```python
from build123d import *

# Parameters (mm, degrees)
EXTRUDE_373_DEPTH      = 12.5
SKETCH_4_W             = 0.8
SKETCH_4_H             = 12.320508076
CHAMFER_2074_SIZE      = 2
FILLET_2116_R          = 0.8
PATTERN_LINEAR_1_COUNT = 20
PATTERN_LINEAR_1_PITCH = 2.421052632


with BuildPart() as part:
    # 草图1 → Extrude 373 (new body)
    with BuildSketch(Plane(origin=(0, 0, 0), x_dir=(0, 0, -1), z_dir=(1, 0, 0))):
        Polygon((15, 8.660254038), (15, -8.660254038), (0, -17.320508076), (-15, -8.660254038), (-15, 8.660254038), (0, 17.320508076), align=None)
    extrude(amount=EXTRUDE_373_DEPTH)

    # 草图2 → 凸台-旋转1 (revolve)
    with BuildSketch(Plane.XY, mode=Mode.PRIVATE) as revolve_1_sk:
        Polygon((0, 0), (92.5, 0), (92.5, 7.835), (92.5, 10), (27.8072, 10), (0, 10), align=None)
    revolve(revolve_1_sk.sketch.rotate(Axis((0, 0, 0), (1, 0, 0)), 90), axis=Axis((0, 0, 0), (1, 0, 0)))

    # 草图3 → 切除-旋转1 (revolve, cut)
    with BuildSketch(Plane.XY):
        Polygon((0, 15), (4.226497308, 22.320508076), (4.226497308, 27.320508076), (-10, 27.320508076), (-10, 15), align=None)
    revolve(axis=Axis((0, 0, 0), (1, 0, 0)), mode=Mode.SUBTRACT)

    # 草图5 → 切除-旋转2 (revolve, cut)
    with BuildSketch(Plane.XY):
        Polygon((12.5, 15), (8.273502692, 22.320508076), (8.273502692, 27.320508076), (18.273502692, 27.320508076), (18.273502692, 15), align=None)
    revolve(axis=Axis((0, 0, 0), (1, 0, 0)), mode=Mode.SUBTRACT)

    # 草图4 → 切除-旋转3 (revolve, cut)
    with BuildSketch(Plane.XY, mode=Mode.PRIVATE) as cut_revolve_3_sk:
        with Locations((12.1, 21.160254038)):
            Rectangle(SKETCH_4_W, SKETCH_4_H)
    revolve(cut_revolve_3_sk.sketch.rotate(Axis((0, 0, 0), (1, 0, 0)), 270), axis=Axis((0, 0, 0), (1, 0, 0)), mode=Mode.SUBTRACT)

    # Chamfer 2074
    chamfer_2074_edges = [part.edges().sort_by_distance(p)[0] for p in [
        (92.5, 0, -10),
    ]]
    chamfer(chamfer_2074_edges, length=CHAMFER_2074_SIZE)

    # Fillet 2116
    fillet_2116_edges = [part.edges().sort_by_distance(p)[0] for p in [
        (12.5, 0, -10),
    ]]
    fillet(fillet_2116_edges, radius=FILLET_2116_R)

    # 草图6 → 切除-旋转4 (revolve, cut)
    with BuildSketch(Plane.XY):
        Polygon((46.5, -7.835), (45.250036667, -10), (45.250036667, -12.5), (47.749963333, -12.5), (47.749963333, -10), align=None)
    cut_revolve_4 = revolve(axis=Axis((-3.175, 0, 0), (1, 0, 0)), mode=Mode.SUBTRACT)

    # 阵列(线性)1: 切除-旋转4 ×20
    with Locations(*[(i * PATTERN_LINEAR_1_PITCH, 0, 0) for i in range(1, PATTERN_LINEAR_1_COUNT)]):
        add(cut_revolve_4, mode=Mode.SUBTRACT)


solid = part.part
```
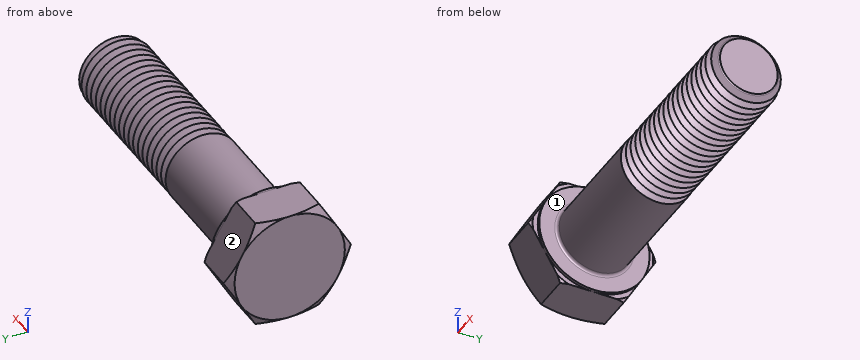
Here's how the part is built. I have some questions about the finished solid (model axes, mm). Face numbers are marked on the shaded views. A direction names the side the tool comes from. Give positions to 0.01 mm unless a question says otherwise; leave off trailing zeros. Loops run counter-clockwise (first coordinate to the right, second up) from the corner with the lowest first, then second, coordinate; pieces in that order, holes last. Notation, with made-up numbers: M 9.25,-14.5 L 35.25,-14.5 A26 ccw 35.25,23.5 Z; hole C -39,4.25 d3. An arc over 180 degrees is marked long. Return JSON: item names as keys, results as strings.
Item 1: Please list where these lines run through material, in increasing order: line 1 (X direction, y = 11, z = 0); line 2 (Y direction, x = 38.5, z = -7.5); line 3 (Z direction, x = 24.5, y = -6).
A:
{"line 1": "x = 0 to 12.5", "line 2": "y = -6.61 to 6.61", "line 3": "z = -8 to 8"}
Item 2: Imagine slicing it at A-A on x = 22. List the corners of the cut face in (y, z) for me.
A:
{"outline": "C 0,0 d20"}
Item 3: I'm going to push flat-ended pins straight in: pin 1 Ø2 at (y, z) = (4, -10) entering from +X; pin 2 Ø1.5 at (x, y) = (42, 10) entering from +Z; pin 3 Ø3.5 at (y, z) = (9, 11.5) entering from +X. Where does each tip first touch, or does it pass through?
A:
{"pin 1": "stops at x = 88.96", "pin 2": "stops at z = 3.8", "pin 3": "stops at x = 12.5"}
Item 4: On a 3-axis mill with a long thin cutter (end or side, diameter ignored), from which of +Z, -Z, +X, -X, +Y, -Y can I reach the whole of each face in a straight line? I mean the marked faces 1 and 2. Say none if no direction works.
A:
{"face 1": "+X", "face 2": "+Z, +X, -X, +Y"}
